For this review, take the finished solid that the model builds, in its own axes (mm). Face numbers are marked on the shaded views. Coordinates: 2 decimals unless noted, no trailing zeros. Loops run counter-clockwise (first coordinate to the right, second up) from the corner with the lowest first, then second, coordinate; pieces in that order, holes last. Notation, with made-up numbers: M 62.25,50.5 L 77.25,50.5 A12 cw 77.25,70.5 Z; hole C 36,26 d11. An arc over 180 degrees is marked long. Write item = value, one per line.
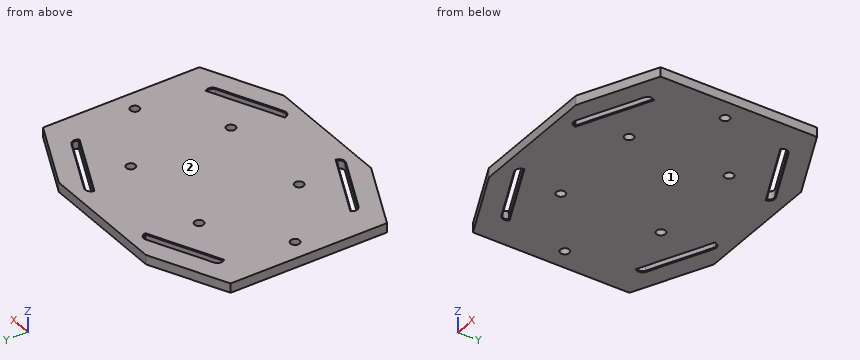
from build123d import *

# Parameters (mm, degrees)
SKETCH3_R           = 4.572
BOSS_EXTRUDE1_DEPTH = 9.525
FILLET1_R           = 4.92
FILLET2_R           = 4.92
CHAMFER1_SIZE       = 0.762
CHAMFER2_SIZE       = 0.762
FILLET3_R           = 4.92
FILLET4_R           = 4.92
FILLET5_R           = 4.92
FILLET6_R           = 4.92
FILLET7_R           = 4.92
FILLET8_R           = 4.92
CHAMFER3_SIZE       = 0.762
CHAMFER4_SIZE       = 0.762
CHAMFER5_SIZE       = 0.762


with BuildPart() as part:
    # Sketch3 → Boss-Extrude1 (new body)
    with BuildSketch(Plane.XY):
        Polygon((64.86807053, -114.3), (-64.86807053, -114.3), (-139.7, -79.405298214), (-139.7, 79.405298214), (-64.86807053, 114.3), (64.86807053, 114.3), (139.7, 79.405298214), (139.7, -79.405298214), align=None)
        with Locations(Location((-50.8, 50.8, 0), (0, 0, 180))):
            Circle(SKETCH3_R, mode=Mode.SUBTRACT)
        with Locations(Location((50.8, 50.8, 0), (0, 0, 180))):
            Circle(SKETCH3_R, mode=Mode.SUBTRACT)
        with Locations(Location((50.8, -50.8, 0), (0, 0, 180))):
            Circle(SKETCH3_R, mode=Mode.SUBTRACT)
        with Locations(Location((-50.8, -50.8, 0), (0, 0, 180))):
            Circle(SKETCH3_R, mode=Mode.SUBTRACT)
        with Locations(Location((-119.38, 0, 0), (0, 0, 180))):
            Circle(SKETCH3_R, mode=Mode.SUBTRACT)
        with Locations(Location((119.38, 0, 0), (0, 0, 180))):
            Circle(SKETCH3_R, mode=Mode.SUBTRACT)
        Polygon((-107.675595872, 64.911434008), (-38.6149425, 97.114945552), (-41.298568462, 102.87), (-110.359221834, 70.666488455), align=None, mode=Mode.SUBTRACT)
        Polygon((38.6149425, 97.114945552), (41.298568462, 102.87), (110.359221834, 70.666488455), (107.675595872, 64.911434008), align=None, mode=Mode.SUBTRACT)
        Polygon((-38.6149425, -97.114945552), (-41.298568462, -102.87), (-110.359221834, -70.666488455), (-107.675595872, -64.911434008), align=None, mode=Mode.SUBTRACT)
        Polygon((107.675595872, -64.911434008), (38.6149425, -97.114945552), (41.298568462, -102.87), (110.359221834, -70.666488455), align=None, mode=Mode.SUBTRACT)
    extrude(amount=BOSS_EXTRUDE1_DEPTH)

    # Fillet1
    fillet1_edges = [part.edges().sort_by_distance(p)[0] for p in [
        (-41.298568462, 102.87, 4.7625),
    ]]
    fillet(fillet1_edges, radius=FILLET1_R)

    # Fillet2
    fillet2_edges = [part.edges().sort_by_distance(p)[0] for p in [
        (-110.359221834, 70.666488455, 4.7625),
    ]]
    fillet(fillet2_edges, radius=FILLET2_R)

    # Chamfer1
    chamfer1_edges = [part.edges().sort_by_distance(p)[0] for p in [
        (-75.828895148, 86.768244228, 9.525),
        (-41.995581821, 100.954971534, 9.525),
        (-107.977767929, 65.559444075, 9.525),
        (-108.444193368, 69.969475096, 9.525),
        (-73.145269186, 81.01318978, 9.525),
        (-38.917114557, 97.76295562, 9.525),
    ]]
    chamfer(chamfer1_edges, length=CHAMFER1_SIZE)

    # Chamfer2
    chamfer2_edges = [part.edges().sort_by_distance(p)[0] for p in [
        (-75.828895148, 86.768244228, 0),
        (-41.995581821, 100.954971534, 0),
        (-107.977767929, 65.559444075, 0),
        (-108.444193368, 69.969475096, 0),
        (-73.145269186, 81.01318978, 0),
        (-38.917114557, 97.76295562, 0),
    ]]
    chamfer(chamfer2_edges, length=CHAMFER2_SIZE)

    # Fillet3
    fillet3_edges = [part.edges().sort_by_distance(p)[0] for p in [
        (41.298568462, 102.87, 4.7625),
    ]]
    fillet(fillet3_edges, radius=FILLET3_R)

    # Fillet4
    fillet4_edges = [part.edges().sort_by_distance(p)[0] for p in [
        (110.359221834, 70.666488455, 4.7625),
    ]]
    fillet(fillet4_edges, radius=FILLET4_R)

    # Fillet5
    fillet5_edges = [part.edges().sort_by_distance(p)[0] for p in [
        (110.359221834, -70.666488455, 4.7625),
    ]]
    fillet(fillet5_edges, radius=FILLET5_R)

    # Fillet6
    fillet6_edges = [part.edges().sort_by_distance(p)[0] for p in [
        (41.298568462, -102.87, 4.7625),
    ]]
    fillet(fillet6_edges, radius=FILLET6_R)

    # Fillet7
    fillet7_edges = [part.edges().sort_by_distance(p)[0] for p in [
        (-41.298568462, -102.87, 4.7625),
    ]]
    fillet(fillet7_edges, radius=FILLET7_R)

    # Fillet8
    fillet8_edges = [part.edges().sort_by_distance(p)[0] for p in [
        (-110.359221834, -70.666488455, 4.7625),
    ]]
    fillet(fillet8_edges, radius=FILLET8_R)

    # Chamfer3
    chamfer3_edges = [part.edges().sort_by_distance(p)[0] for p in [
        (38.917114557, 97.76295562, 0),
        (38.917114557, 97.76295562, 9.525),
        (41.995581821, 100.954971534, 0),
        (41.995581821, 100.954971534, 9.525),
        (75.828895148, 86.768244228, 9.525),
        (75.828895148, 86.768244228, 0),
        (108.444193368, 69.969475096, 0),
        (108.444193368, 69.969475096, 9.525),
        (73.145269186, 81.01318978, 0),
        (107.977767929, 65.559444075, 0),
        (73.145269186, 81.01318978, 9.525),
        (107.977767929, 65.559444075, 9.525),
    ]]
    chamfer(chamfer3_edges, length=CHAMFER3_SIZE)

    # Chamfer4
    chamfer4_edges = [part.edges().sort_by_distance(p)[0] for p in [
        (-38.917114557, -97.76295562, 0),
        (-38.917114557, -97.76295562, 9.525),
        (-41.995581821, -100.954971534, 0),
        (-41.995581821, -100.954971534, 9.525),
        (-75.828895148, -86.768244228, 9.525),
        (-75.828895148, -86.768244228, 0),
        (-108.444193368, -69.969475096, 9.525),
        (-108.444193368, -69.969475096, 0),
        (-73.145269186, -81.01318978, 0),
        (-107.977767929, -65.559444075, 0),
        (-73.145269186, -81.01318978, 9.525),
        (-107.977767929, -65.559444075, 9.525),
    ]]
    chamfer(chamfer4_edges, length=CHAMFER4_SIZE)

    # Chamfer5
    chamfer5_edges = [part.edges().sort_by_distance(p)[0] for p in [
        (107.977767929, -65.559444075, 0),
        (107.977767929, -65.559444075, 9.525),
        (108.444193368, -69.969475096, 0),
        (108.444193368, -69.969475096, 9.525),
        (75.828895148, -86.768244228, 9.525),
        (75.828895148, -86.768244228, 0),
        (41.995581821, -100.954971534, 9.525),
        (41.995581821, -100.954971534, 0),
        (73.145269186, -81.01318978, 0),
        (38.917114557, -97.76295562, 0),
        (73.145269186, -81.01318978, 9.525),
        (38.917114557, -97.76295562, 9.525),
    ]]
    chamfer(chamfer5_edges, length=CHAMFER5_SIZE)


solid = part.part
Q1. Add section D-D (z = 6.25). State how many separate pieces and enclosed holes the cut face has, and give its area (3 significant figures).
Solved:
separate_pieces = 1
enclosed_holes = 10
area = 56,400 mm²
Q2. Draft analysis for pull direction Z (two halves, no side actions). For the marked faces 1 and 2, state which applies: +Z half, -Z half, draft (parallel to the pull), parting line (faces both ways), or undercut.
Solved:
face_1 = -Z half
face_2 = +Z half
Q3. Add section A-A (y = 0). Write out the cut boundary in (x, z) (3 decimals), and give its area (3 significant figures).
Solved:
outline = M -139.7,0 L -123.952,0 L -123.952,9.525 L -139.7,9.525 Z; M -114.808,0 L 114.808,0 L 114.808,9.525 L -114.808,9.525 Z; M 123.952,0 L 139.7,0 L 139.7,9.525 L 123.952,9.525 Z
area = 2,490 mm²
Q4. Add section B-B (x = 50.8). Write out the cut boundary in (y, z) (3 decimals), and give its area (3 significant figures).
Solved:
outline = M -114.3,0 L -99.28,0 L -98.439,0.762 L -98.439,8.763 L -99.28,9.525 L -114.3,9.525 Z; M -91.433,0.762 L -90.592,0 L -55.372,0 L -55.372,9.525 L -90.592,9.525 L -91.433,8.763 Z; M -46.228,0 L 46.228,0 L 46.228,9.525 L -46.228,9.525 Z; M 55.372,0 L 90.592,0 L 91.433,0.762 L 91.433,8.763 L 90.592,9.525 L 55.372,9.525 Z; M 98.439,0.762 L 99.28,0 L 114.3,0 L 114.3,9.525 L 99.28,9.525 L 98.439,8.763 Z
area = 1,870 mm²
Q5. For line 1 along X through (y, z) = (50.8, 4); line 2 along Y through (x, z) = (82.5, 7.5); line 3 along Y through (x, z) = (52.5, 3.5), list the stretches that pass through material, from the lowest coordinate up.
Solved:
line_1 = -139.7 to -55.37, -46.23 to 46.23, 55.37 to 139.7
line_2 = -106.08 to -83.66, -76.65 to 76.65, 83.66 to 106.08
line_3 = -114.3 to -97.65, -90.64 to -55.04, -46.56 to 46.56, 55.04 to 90.64, 97.65 to 114.3
Q6. Add section C-C (x = -119). Write out the cut boundary in (y, z) (3 decimals), and give its area (3 significant figures).
Solved:
outline = M -89.058,0 L -4.556,0 L -4.556,9.525 L -89.058,9.525 Z; M 4.556,0 L 89.058,0 L 89.058,9.525 L 4.556,9.525 Z
area = 1,610 mm²
Q7. For pin 1 Ø5.5 at (x, y) = (-119.38, 0) entering from -Z; pin 2 Ø5 at (x, z) = (-69.5, 4) entering from -Y, all flat-tipped, find the tip position at first contact; note any pin that passes through.
Solved:
pin_1 = through
pin_2 = -113.31
